from build123d import *

# Parameters (mm, degrees)
F1_DEPTH = 12


with BuildPart() as f1:
    # F0 (on Top) → F1 (new body)
    with BuildSketch(Plane.XY):
        with BuildLine():
            ThreePointArc((28, 0), (25.071068, 7.071068), (18, 10))
            Line((18, 10), (-18, 10))
            ThreePointArc((-18, 10), (-25.071068, 7.071068), (-28, 0))
            ThreePointArc((-28, 0), (-25.071068, -7.071068), (-18, -10))
            Line((-18, -10), (18, -10))
            ThreePointArc((18, -10), (25.071068, -7.071068), (28, 0))
        make_face()
    extrude(amount=F1_DEPTH)


solid = f1.part
Source: CAD feature listing. Evaluate the final solid. Frame: model axes, mm. Round coordinates to 2 decimals unless told otherwise and drop trailing zeros. Loops run counter-clockwise (first coordinate to the right, second up) from the corner with the lowest first, then second, coordinate; pieces in that order, holes last.
Q1. Section B-B, the plane y = 6. Return loops of the section in (x, z).
Q2. Section C-C, the plane y = 8.5. Return loops of the section in (x, z).
Q3. Ray query, line 1 (X direction, y = 8.75, z = 9.75); line 2 (X direction, y = 7, z = 5.5); line 3 (Y direction, x = -26, z = 11.5). Return the intervals inside material, ascending.
Q4. Section A-A, the plane z = 7.5. Return loops of the section in (x, y).
Q5. First-contact query: P1, Ø5, axis at y = 7.5, z = 1.5, coming from the +X side; P2, Ø3, axis at y = 4.5, z = 7.5, coming from the +X side; P3, Ø3, axis at y = 7, z = 10, coming from the -X side. Flat tips, straight axial feed; report the tip coordinate or a pass-through.
Solutions:
1. outline: (-26, 0) - (26, 0) - (26, 12) - (-26, 12) - close
2. outline: (-23.27, 0) - (23.27, 0) - (23.27, 12) - (-23.27, 12) - close
3. line 1: x = -22.84 to 22.84
3. line 2: x = -25.14 to 25.14
3. line 3: y = -6 to 6
4. outline: (-28, 0) arc R10 ccw to (-18, -10) - (18, -10) arc R10 ccw to (28, 0) arc R10 ccw to (18, 10) - (-18, 10) arc R10 ccw to start
5. P1: stops at x = 26.66
5. P2: stops at x = 27.54
5. P3: stops at x = -26.35
